from build123d import *

# Parameters (mm, degrees)
BASE_FLANGE1_START           = -3.4
BASE_FLANGE1_OUTLINE_R       = 17.5
BASE_FLANGE1_DEPTH           = 3.4
EDGE_FLANGE2_STRIP_W         = 15.0732
EDGE_FLANGE2_STRIP_H         = 3.4
EDGE_FLANGE2_STRIP_CUT_DEPTH = 92.6
EDGE_FLANGE2_DEPTH           = 92.6
EDGE_FLANGE2_PROFILE_W       = 92.6
EDGE_FLANGE2_PROFILE_H       = 75.8634
EDGE_FLANGE2_PROFILE_R       = 5
EDGE_FLANGE2_FLAT_DEPTH      = 3.4
EDGE_FLANGE3_STRIP_W         = 15.0732
EDGE_FLANGE3_STRIP_H         = 3.4
EDGE_FLANGE3_STRIP_CUT_DEPTH = 92.6
EDGE_FLANGE3_DEPTH           = 92.6
EDGE_FLANGE3_PROFILE_W       = 92.6
EDGE_FLANGE3_PROFILE_H       = 75.8634
EDGE_FLANGE3_PROFILE_R       = 5
EDGE_FLANGE3_FLAT_DEPTH      = 3.4


# Read off the part's stored shape, not the designer's step: Base-Flange1
# Sheet-metal steps are written as plain solids
with BuildPart() as part:
    # Base-Flange1 outline → Base-Flange1 (new body)
    with BuildSketch(Plane.XY.offset(BASE_FLANGE1_START)):
        with BuildLine():
            Line((0, -92.6), (0, 0))
            Line((0, 0), (-288.2, 0))
            Line((-288.2, 0), (-288.2, -92.6))
            Line((-288.2, -92.6), (-273.2, -92.6))
            ThreePointArc((-273.2, -92.6), (-271.814311921, -88.29213457), (-268.176971207, -85.6))
            Line((-268.176971207, -85.6), (-20.023028793, -85.6))
            ThreePointArc((-20.023028793, -85.6), (-16.385688079, -88.29213457), (-15, -92.6))
            Line((-15, -92.6), (0, -92.6))
        make_face()
        with Locations((-245.7, -46.3)):
            Circle(BASE_FLANGE1_OUTLINE_R, mode=Mode.SUBTRACT)
        with Locations((-196.483203415, -46.3)):
            Circle(BASE_FLANGE1_OUTLINE_R, mode=Mode.SUBTRACT)
        with Locations((-144.1, -42.8)):
            Circle(BASE_FLANGE1_OUTLINE_R, mode=Mode.SUBTRACT)
        with Locations((-91.716796585, -46.3)):
            Circle(BASE_FLANGE1_OUTLINE_R, mode=Mode.SUBTRACT)
        with Locations((-42.5, -46.3)):
            Circle(BASE_FLANGE1_OUTLINE_R, mode=Mode.SUBTRACT)
    extrude(amount=BASE_FLANGE1_DEPTH)

    # Edge-Flange2 strip (across the edge) → Edge-Flange2 strip cut (cut)
    with BuildSketch(Plane(origin=(-288.2, 0, 0), x_dir=(1, 0, 0), z_dir=(0, -1, 0))):
        with Locations((-3.4, -1.7)):
            Rectangle(EDGE_FLANGE2_STRIP_W, EDGE_FLANGE2_STRIP_H)
    extrude(amount=EDGE_FLANGE2_STRIP_CUT_DEPTH, mode=Mode.SUBTRACT)

    # Edge-Flange2 bend section (across the edge) → Edge-Flange2 (add)
    with BuildSketch(Plane(origin=(-288.2, 0, 0), x_dir=(1, 0, 0), z_dir=(0, -1, 0))):
        with BuildLine():
            Line((0, 0.7366), (3.4, 0.7366))
            ThreePointArc((3.4, 0.7366), (3.615745145, 0.215745145), (4.1366, 0))
            Line((4.1366, 0), (4.1366, -3.4))
            ThreePointArc((4.1366, -3.4), (1.211582089, -2.188417911), (0, 0.7366))
        make_face()
    extrude(amount=EDGE_FLANGE2_DEPTH)

    # Edge-Flange2 profile (on flange) → Edge-Flange2 flat (add)
    with BuildSketch(Plane.YZ.offset(-288.2)):
        with Locations((-46.3, 38.6683)):
            Rectangle(EDGE_FLANGE2_PROFILE_W, EDGE_FLANGE2_PROFILE_H)
        with Locations((-29.7, 28.6)):
            Circle(EDGE_FLANGE2_PROFILE_R, mode=Mode.SUBTRACT)
        with Locations((-69.7, 28.6)):
            Circle(EDGE_FLANGE2_PROFILE_R, mode=Mode.SUBTRACT)
    extrude(amount=EDGE_FLANGE2_FLAT_DEPTH)

    # Edge-Flange3 strip (across the edge) → Edge-Flange3 strip cut (cut)
    with BuildSketch(Plane(origin=(0, -92.6, 0), x_dir=(-1, 0, 0), z_dir=(0, 1, 0))):
        with Locations((-3.4, -1.7)):
            Rectangle(EDGE_FLANGE3_STRIP_W, EDGE_FLANGE3_STRIP_H)
    extrude(amount=EDGE_FLANGE3_STRIP_CUT_DEPTH, mode=Mode.SUBTRACT)

    # Edge-Flange3 bend section (across the edge) → Edge-Flange3 (add)
    with BuildSketch(Plane(origin=(0, -92.6, 0), x_dir=(-1, 0, 0), z_dir=(0, 1, 0))):
        with BuildLine():
            Line((0, 0.7366), (3.4, 0.7366))
            ThreePointArc((3.4, 0.7366), (3.615745145, 0.215745145), (4.1366, 0))
            Line((4.1366, 0), (4.1366, -3.4))
            ThreePointArc((4.1366, -3.4), (1.211582089, -2.188417911), (0, 0.7366))
        make_face()
    extrude(amount=EDGE_FLANGE3_DEPTH)

    # Edge-Flange3 profile (on flange) → Edge-Flange3 flat (add)
    with BuildSketch(Plane.YZ):
        with Locations((-46.3, 38.6683)):
            Rectangle(EDGE_FLANGE3_PROFILE_W, EDGE_FLANGE3_PROFILE_H)
        with Locations((-69.7, 28.6)):
            Circle(EDGE_FLANGE3_PROFILE_R, mode=Mode.SUBTRACT)
        with Locations((-29.7, 28.6)):
            Circle(EDGE_FLANGE3_PROFILE_R, mode=Mode.SUBTRACT)
    extrude(amount=-EDGE_FLANGE3_FLAT_DEPTH)


solid = part.part
CAD build for the part. Positions are in the model's coordinates, mm. A direction names the side the tool comes from. Coordinates: 2 decimals unless noted, no trailing zeros. Write each loop counter-clockwise with the first axis right and the second up, starting at its lowest first coordinate (ties: lowest second). Pieces come first, ordered by that corner, then holes. Notation, with made-up numbers: (-11.75, 8.25) - (0.25, 8.25) arc R7 cw to (0.25, 12.25) - close; hole circle Ø1 at (11, 71.5). An arc over 180 degrees is marked (long way). Use a Markdown table: item, result. Add a question column.
Item 1: Flat gauge pins, fed straight in: pin 1 (8 mm diameter, centred on x = -55.5, y = -63, fed in from +Z); pin 2 (2.5 mm diameter, centred on x = -163, z = -1.5, fed in from -Y). Where does each tip first touch, or does it go through?
Item 2: Band-saw the part on D-D, the plane z = 28.6. Give the cut face in (x, y), and give its area (3 significant figures).
Item 3: Drill centre lines: L1, parallel to X at y = -84.5, z = 7.5; L2, parallel to Y at x = -285, z = 28; L3, parallel to Z at x = -39, y = -74. Where is each one in solid material? Low to high. Write a range as from..to.
Item 4: Band-saw the part on A-A, the plane z = 69.5. Give the cut face in (x, y).
Item 5: 3-axis set-ups, long thin cutter, end or side, ignore diameter. For faces 1 (the face through (-16.423, -88.24, -1.724)), 2 (the face through (-284.8, -47, 39)), 3 (the face through (-285, -92.6, 33)): which of +Z, -Z, +X, -X, +Y, -Y reach the whole face in a straight line?
Item 6: Band-saw the part on B-B, the plane y = -69.7. Give the cut face in (x, z), and give its area (3 significant figures).
Item 7: Mould opens along X. For faces 4 (the face through (-210.37, -56.95, -1.72)), 5 (the face through (0, -47, 39)), 6 (the face through (-286.52, -64.93, 30.1)), 7 (the face through (-288.2, -47, 39)) say: pulls with the +X half, pulls with the -X half, needs draft (parallel to the pull), parting line crosses it, or undercut.
Item 8: Band-saw the part on C-C, the plane x = -245.7. Give the cut face in (y, z), and give its area (3 significant figures).
Numbers:
| question | item | result |
|---|---|---|
| 1 | pin 1 | z = 0 |
| 1 | pin 2 | y = -85.6 |
| 2 | outline | (-288.2, -92.6) - (-284.8, -92.6) - (-284.8, -74.7) - (-288.2, -74.7) - close; (-288.2, -64.7) - (-284.8, -64.7) - (-284.8, -34.7) - (-288.2, -34.7) - close; (-288.2, -24.7) - (-284.8, -24.7) - (-284.8, 0) - (-288.2, 0) - close; (-3.4, -92.6) - (0, -92.6) - (0, -74.7) - (-3.4, -74.7) - close; (-3.4, -64.7) - (0, -64.7) - (0, -34.7) - (-3.4, -34.7) - close; (-3.4, -24.7) - (0, -24.7) - (0, 0) - (-3.4, 0) - close |
| 2 | area | 494 mm2 |
| 3 | L1 | -288.2..-284.8, -3.4..0 |
| 3 | L2 | -92.6..-74.66, -64.74..-34.66, -24.74..0 |
| 3 | L3 | -3.4..0 |
| 4 | outline | (-288.2, -92.6) - (-284.8, -92.6) - (-284.8, 0) - (-288.2, 0) - close; (-3.4, -92.6) - (0, -92.6) - (0, 0) - (-3.4, 0) - close |
| 5 | face 1 | +Z, -Z, -Y |
| 5 | face 2 | +Z, +Y, -Y |
| 5 | face 3 | +Z, -Z, +X, -X, -Y |
| 6 | outline | (-288.2, 0.74) arc R4.14 ccw to (-284.06, -3.4) - (-4.14, -3.4) arc R4.14 ccw to (0, 0.74) - (0, 23.6) - (-3.4, 23.6) - (-3.4, 0.74) arc R0.74 cw to (-4.14, 0) - (-284.06, 0) arc R0.74 cw to (-284.8, 0.74) - (-284.8, 23.6) - (-288.2, 23.6) - close; (-288.2, 33.6) - (-284.8, 33.6) - (-284.8, 76.6) - (-288.2, 76.6) - close; (-3.4, 33.6) - (0, 33.6) - (0, 76.6) - (-3.4, 76.6) - close |
| 6 | area | 1,430 mm2 |
| 7 | face 4 | undercut |
| 7 | face 5 | pulls with the +X half |
| 7 | face 6 | needs draft |
| 7 | face 7 | pulls with the -X half |
| 8 | outline | (-85.6, -3.4) - (-63.8, -3.4) - (-63.8, 0) - (-85.6, 0) - close; (-28.8, -3.4) - (0, -3.4) - (0, 0) - (-28.8, 0) - close |
| 8 | area | 172 mm2 |
